from build123d import *

# Parameters (mm, degrees)
SKETCH_R     = 2.75
PAD_DEPTH    = 2
SKETCH001_R  = 1.2
PAD001_DEPTH = 5
FILLET_R     = 1


with BuildPart() as part:
    # Sketch → Pad (new body)
    with BuildSketch(Plane.XY):
        Circle(SKETCH_R)
    extrude(amount=PAD_DEPTH)

    # Sketch001 (on Face3 of Pad) → Pad001 (join)
    with BuildSketch(Plane.XY.offset(2)):
        Circle(SKETCH001_R)
    extrude(amount=PAD001_DEPTH)

    # Fillet
    fillet_edges = [part.edges().sort_by_distance(p)[0] for p in [
        (-1.2, 0, 7),
    ]]
    fillet(fillet_edges, radius=FILLET_R)


solid = part.part
The listing builds one solid part. Answer for the finished solid, in the listing's coordinates (mm). A direction names the side the tool comes from. Give positions to 0.01 mm unless a question says otherwise; leave off trailing zeros. Write each loop counter-clockwise with the first axis right and the second up, starting at its lowest first coordinate (ties: lowest second). Pieces come first, ordered by that corner, then holes. Notation, with made-up numbers: (83, 62.25) -> (130, 62.25) arc R20 ccw to (130, 93.25) -> close; hole circle Ø10 at (-32, -30). An arc over 180 degrees is marked (long way). One line per question, with ' | ' between items. Start each with the question number.
1. Find the intervals of material crossed by probe 1 along Z at (x, y) = (0.45, -2.5); probe 2 along X at (y, z) = (-0.7, 6.75); probe 3 along Y at (x, z) = (-0.4, 3.5), in increasing order.
2. Section C-C (x = 1.35) is taken. Determine the outline of the cut face in (y, z).
3. Given pin 1 Ø1.5 at (x, z) = (0.5, 3) entering from -Y; pin 2 Ø1 at (y, z) = (-1.5, 1) entering from +X; pin 3 Ø2 at (y, z) = (0, 6) entering from -X, each flat-ended and moving along its own axis, determine where each tip first touches the part or whether it passes through.
4. For faces 1 (the cylindrical face through (0.65, 1.01, 3.97)), 2 (the cylindrical face through (-0.596, -2.685, 0.986)), determine the directions among +Z, -Z, +X, -X, +Y, -Y from which every point of the face is accessible in a straight line to the end or side of a thin tool.
5. Section A-A (z = 5.75) is taken. Determine the outline of the cut face in (x, y), plus the area to 3 significant figures.
6. Section B-B (y = -1.8) is taken. Determine the outline of the cut face in (x, z), plus the area to 3 significant figures.
Response values:
1) probe 1: 0 to 2 | probe 2: -0.5 to 0.5 | probe 3: -1.13 to 1.13
2) outline: (-2.4, 0) -> (2.4, 0) -> (2.4, 2) -> (-2.4, 2) -> close
3) pin 1: y = -1.2 | pin 2: x = 2.56 | pin 3: x = -1.2
4) face 1: +Z | face 2: +Z, -Z
5) outline: circle Ø2.4 at (0, 0) | area: 4.52 mm2
6) outline: (-2.08, 0) -> (2.08, 0) -> (2.08, 2) -> (-2.08, 2) -> close | area: 8.32 mm2
